```python
from build123d import *

# Parameters (mm, degrees)
CROQUIS1_R              = 5.25
CROQUIS1_R_2            = 6.75
CROQUIS1_R_3            = 2
CROQUIS1_R_4            = 1.5
CROQUIS1_W              = 6.1
CROQUIS1_H              = 15
SALIENTE_EXTRUIR1_DEPTH = 6


with BuildPart() as part:
    # Croquis1 → Saliente-Extruir1 (new body)
    with BuildSketch(Plane(origin=(0, 0, 0), x_dir=(1, 0, 0), z_dir=(0, 1, 0))):
        with BuildLine():
            Line((16.282727366, 43.644609037), (71.802987861, 43.644609037))
            Line((71.802987861, 43.644609037), (93.167350191, 43.644609037))
            ThreePointArc((93.167350191, 43.644609037), (94.581563754, 43.058822599), (95.167350191, 41.644609037))
            Line((95.167350191, 41.644609037), (95.167350191, 11.644653108))
            ThreePointArc((95.167350191, 11.644653108), (96.557023393, -0.870818798), (100.658344058, -12.7765904))
            ThreePointArc((100.658344058, -12.7765904), (100.070791822, -22.404752266), (91.620792474, -27.057088195))
            Line((91.620792474, -27.057088195), (-122.960915675, -27.057088195))
            ThreePointArc((-122.960915675, -27.057088195), (-131.47488844, -22.30230199), (-131.892437156, -12.559541748))
            ThreePointArc((-131.892437156, -12.559541748), (-127.777809493, -0.78872644), (-126.832649809, 11.644653108))
            Line((-126.832649809, 11.644653108), (-126.832649809, 41.644609037))
            ThreePointArc((-126.832649809, 41.644609037), (-126.246863371, 43.058822599), (-124.832649809, 43.644609037))
            Line((-124.832649809, 43.644609037), (-103.468287478, 43.644609037))
            Line((-103.468287478, 43.644609037), (-60.497048313, 43.644609037))
            Line((-60.497048313, 43.644609037), (-47.948026983, 43.644609037))
            ThreePointArc((-47.948026983, 43.644609037), (-46.533813421, 43.058822599), (-45.948026983, 41.644609037))
            Line((-45.948026983, 41.644609037), (-45.948026983, 38.554619052))
            Line((-45.948026983, 38.554619052), (14.282727366, 38.554619052))
            Line((14.282727366, 38.554619052), (14.282727366, 41.644609037))
            ThreePointArc((14.282727366, 41.644609037), (14.868513803, 43.058822599), (16.282727366, 43.644609037))
        make_face()
        with Locations(Location((-15.832649809, 27.644609037, 0), (0, 0, 270))):
            Circle(CROQUIS1_R, mode=Mode.SUBTRACT)
        with Locations(Location((-110.832649809, 27.644609037, 0), (0, 0, 270))):
            Circle(CROQUIS1_R_2, mode=Mode.SUBTRACT)
        with Locations(Location((79.167350191, 27.644609037, 0), (0, 0, 270))):
            Circle(CROQUIS1_R_2, mode=Mode.SUBTRACT)
        with Locations(Location((-99.51894131, 38.958317536, 0), (0, 0, 270))):
            Circle(CROQUIS1_R_3, mode=Mode.SUBTRACT)
        with Locations(Location((-122.146358308, 38.958317536, 0), (0, 0, 270))):
            Circle(CROQUIS1_R_3, mode=Mode.SUBTRACT)
        with Locations(Location((-99.51894131, 16.330900538, 0), (0, 0, 270))):
            Circle(CROQUIS1_R_3, mode=Mode.SUBTRACT)
        with Locations(Location((-122.146358308, 16.330900538, 0), (0, 0, 270))):
            Circle(CROQUIS1_R_3, mode=Mode.SUBTRACT)
        with Locations(Location((90.48105869, 16.330900538, 0), (0, 0, 270))):
            Circle(CROQUIS1_R_3, mode=Mode.SUBTRACT)
        with Locations(Location((67.853641692, 16.330900538, 0), (0, 0, 270))):
            Circle(CROQUIS1_R_3, mode=Mode.SUBTRACT)
        with Locations(Location((67.853641692, 38.958317536, 0), (0, 0, 270))):
            Circle(CROQUIS1_R_3, mode=Mode.SUBTRACT)
        with Locations(Location((-10.175795559, 33.301463286, 0), (0, 0, 270))):
            Circle(CROQUIS1_R_4, mode=Mode.SUBTRACT)
        with Locations(Location((-21.489504058, 33.301463286, 0), (0, 0, 270))):
            Circle(CROQUIS1_R_4, mode=Mode.SUBTRACT)
        with Locations(Location((-21.489504058, 21.987754787, 0), (0, 0, 270))):
            Circle(CROQUIS1_R_4, mode=Mode.SUBTRACT)
        with Locations(Location((-10.175795559, 21.987754787, 0), (0, 0, 270))):
            Circle(CROQUIS1_R_4, mode=Mode.SUBTRACT)
        with Locations(Location((-110.832649809, 1.644609037, 0), (0, 0, 270))):
            Circle(CROQUIS1_R_4, mode=Mode.SUBTRACT)
        with Locations(Location((79.167361237, 1.644649397, 0), (0, 0, 270))):
            Circle(CROQUIS1_R_4, mode=Mode.SUBTRACT)
        with Locations(Location((90.48105869, 38.958317536, 0), (0, 0, 270))):
            Circle(CROQUIS1_R_3, mode=Mode.SUBTRACT)
        with Locations(Location((-15.828049724, 1.644627362, 0), (0, 0, 270))):
            Circle(CROQUIS1_R_4, mode=Mode.SUBTRACT)
        with Locations((-110.832649809, -13.855390963)):
            Rectangle(CROQUIS1_W, CROQUIS1_H, mode=Mode.SUBTRACT)
        Polygon((76.117364636, -6.355351899), (76.117371009, -21.355351899), (82.217371009, -21.355349308), (82.217364636, -6.355349308), align=None, mode=Mode.SUBTRACT)
        Polygon((-18.88264641, -6.355351899), (-18.882640037, -21.355351899), (-12.782640037, -21.355349308), (-12.78264641, -6.355349308), align=None, mode=Mode.SUBTRACT)
    extrude(amount=SALIENTE_EXTRUIR1_DEPTH)


solid = part.part
```
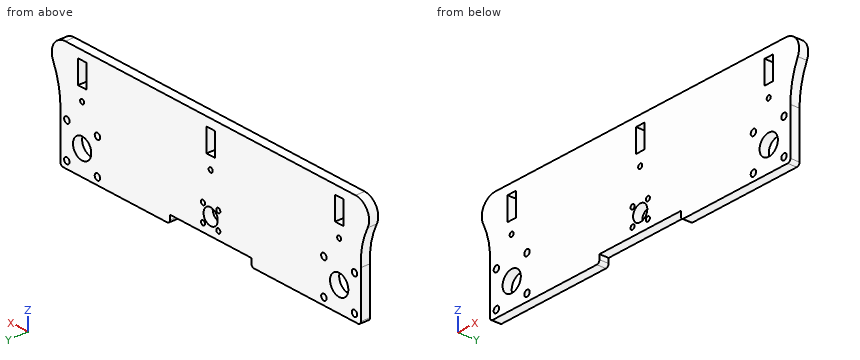
Design review of the part built by this model. Coordinates are the model's own, in mm. Coordinates: 2 decimals unless noted, no trailing zeros. Write each loop counter-clockwise with the first axis right and the second up, starting at its lowest first coordinate (ties: lowest second). Pieces come first, ordered by that corner, then holes. Notation, with made-up numbers: M -30,70.5 L 7,70.5 A33 cw 7,98.5 Z; hole C -28,80 d5. An arc over 180 degrees is marked long. Answer as a JSON object with one key per item and string values.
Item 1: Add section D-D, the plane z = 3. Give the boundary of the cut face in (x, y), and give its area (3 significant figures).
Outcome:
{"outline": "M -128.29,0 L 97.08,0 L 97.08,6 L -128.29,6 Z", "area": "1,350 mm²"}
Item 2: Add section C-C, the plane y = 2.8. State how many separate pieces and enclosed holes the cut face has, and give its area (3 significant figures).
Outcome:
{"separate pieces": "1", "enclosed holes": "21", "area": "14,800 mm²"}
Item 3: Add section A-A, the plane z = -26. Give the boundary of the cut face in (x, y).
Outcome:
{"outline": "M -126.83,0 L -117.38,0 L -117.38,6 L -126.83,6 Z; M -104.29,0 L -20.82,0 L -20.82,6 L -104.29,6 Z; M -10.85,0 L 72.62,0 L 72.62,6 L -10.85,6 Z; M 85.71,0 L 95.17,0 L 95.17,6 L 85.71,6 Z"}
Item 4: Add section B-B, the plane z = 15.5. Give the boundary of the cut face in (x, y).
Outcome:
{"outline": "M -132.84,0 L -113.88,0 L -113.88,6 L -132.84,6 Z; M -107.78,0 L -18.88,0 L -18.88,6 L -107.78,6 Z; M -12.78,0 L 76.12,0 L 76.12,6 L -12.78,6 Z; M 82.22,0 L 101.5,0 L 101.5,6 L 82.22,6 Z"}
Item 5: Wall thickness on probe 1 along Z at (x, y) = (-122.5, 3.35); probe 2 along X at (y, z) = (1.8, 17.5); probe 3 along X at (y, z) = (2.45, 12.5): over which ranges is each line inside the solid? List them lowest first.
Outcome:
{"probe 1": "-43.64 to -40.93, -36.99 to -18.3, -14.36 to 27.06", "probe 2": "-132.95 to -113.88, -107.78 to -18.88, -12.78 to 76.12, 82.22 to 101.61", "probe 3": "-131.86 to -113.88, -107.78 to -18.88, -12.78 to 76.12, 82.22 to 100.53"}
Item 6: Insertion check: pin 1 Ø1.5 at (y, z) = (2.5, 19) entering from -X; pin 2 Ø1.8 at (x, z) = (-10.18, -21.99) entering from -Y; pin 3 Ø3.5 at (y, z) = (3, -40) entering from -X; pin 4 Ø1.8 at (y, z) = (3.5, 13.5) entering from -X. Each pin has a flat end and moves straight along its axis. Give the tip position at first contact, or say it passes through.
Outcome:
{"pin 1": "x = -132.89", "pin 2": "through", "pin 3": "x = -126.83", "pin 4": "x = -132.6"}
